Could you check a few things on this model? Use its own coordinates, in mm. A direction names the side the tool comes from. Give positions to 0.01 mm unless a question says otherwise; leave off trailing zeros. Order: outer loops, then holes, each group sorted by start corner. A loop starts at its lowest first (then second) coordinate and runs counter-clockwise, first axis right, second up. Notation, with made-up numbers: (77, 37) - (86, 37) arc R10 cw to (86, 43) - close; hole circle Ø6 at (60.25, -13). An arc over 180 degrees is marked (long way). Put each result on its own line as item: value.
from build123d import *

# Parameters (mm, degrees)
F0_W     = 41.148
F0_H     = 61.214
F1_DEPTH = 1.3
F2_R     = 1
F3_DEPTH = 1.3
F4_DEPTH = 4.5
F2_W     = 10.16
F2_H     = 1.5257
F5_DEPTH = 10.5
F2_H_2   = 4.445
F2_W_2   = 5.08
F6_DEPTH = 3.5
F2_H_3   = 1.905
F7_DEPTH = 11.5
F2_W_3   = 12.7
F8_DEPTH = 7.2


with BuildPart() as f1:
    # F0 (on Top) → F1 (new body)
    with BuildSketch(Plane.XY):
        Rectangle(F0_W, F0_H)
    extrude(amount=F1_DEPTH)

    # F2 (on face) → F3 (cut, through all)
    with BuildSketch(Plane.XY.offset(1.3)):
        with Locations((-18.034, 17.145)):
            Circle(F2_R)
        with Locations((18.034, 27.305)):
            Circle(F2_R)
        with Locations((18.034, -28.575)):
            Circle(F2_R)
    extrude(amount=-F3_DEPTH, mode=Mode.SUBTRACT)

    # F2 (on face) → F4 (join)
    with BuildSketch(Plane.XY.offset(1.3)):
        with BuildLine():
            ThreePointArc((-18.034, -4.826), (-17.399, -5.461), (-18.034, -6.096))
            Line((-18.034, -6.096), (-18.034, -8.255))
            Line((-18.034, -8.255), (19.05, -8.255))
            Line((19.05, -8.255), (19.05, -2.667))
            Line((19.05, -2.667), (-18.034, -2.667))
            Line((-18.034, -2.667), (-18.034, -4.826))
        make_face()
        with BuildLine():
            Line((14.224, 3.556), (14.224, 9.398))
            Line((14.224, 9.398), (-6.096, 9.398))
            Line((-6.096, 9.398), (-6.096, 7.493))
            ThreePointArc((-6.096, 7.493), (-5.08, 6.477), (-6.096, 5.461))
            Line((-6.096, 5.461), (-6.096, 3.556))
            Line((-6.096, 3.556), (14.224, 3.556))
        make_face()
        with BuildLine():
            Line((-1.016, -14.478), (-1.016, -20.32))
            Line((-1.016, -20.32), (19.304, -20.32))
            Line((19.304, -20.32), (19.304, -18.415))
            ThreePointArc((19.304, -18.415), (18.288, -17.399), (19.304, -16.383))
            Line((19.304, -16.383), (19.304, -14.478))
            Line((19.304, -14.478), (-1.016, -14.478))
        make_face()
    extrude(amount=F4_DEPTH)

    # F2 (on face) → F5 (join)
    with BuildSketch(Plane.XY.offset(1.3)):
        with Locations((-12.7211, 28.81415)):
            Rectangle(F2_W, F2_H)
        Polygon((-7.6411, 28.0513), (-17.8011, 28.0513), (-17.8011, 27.5683), (-17.8011, 23.5715), (-17.8011, 23.0791), (-7.6411, 23.0791), (-7.6411, 23.5715), (-7.6411, 27.5683), align=None)
        with BuildLine():
            ThreePointArc((-15.2611, 27.467), (-13.3461, 25.552), (-15.2611, 23.637))
            ThreePointArc((-15.2611, 23.637), (-17.1761, 25.552), (-15.2611, 27.467))
        make_face(mode=Mode.SUBTRACT)
        with BuildLine():
            ThreePointArc((-10.1811, 27.467), (-8.2661, 25.552), (-10.1811, 23.637))
            ThreePointArc((-10.1811, 23.637), (-12.0961, 25.552), (-10.1811, 27.467))
        make_face(mode=Mode.SUBTRACT)
    extrude(amount=F5_DEPTH)

    # F2 (on face) → F6 (join)
    with BuildSketch(Plane.XY.offset(1.3)):
        with Locations((7.874, 24.8285)):
            Rectangle(F2_W, F2_H_2)
        with Locations((-2.54, 17.5895)):
            Rectangle(F2_W_2, F2_H_2)
        with Locations((-13.208, -17.0815)):
            Rectangle(F2_W, F2_H_2)
    extrude(amount=F6_DEPTH)

    # F2 (on face) → F7 (join)
    with BuildSketch(Plane.XY.offset(1.3)):
        with Locations((7.874, 28.0035)):
            Rectangle(F2_W, F2_H_3)
        with Locations((-2.54, 14.4145)):
            Rectangle(F2_W_2, F2_H_3)
        with Locations((-13.208, -13.9065)):
            Rectangle(F2_W, F2_H_3)
    extrude(amount=F7_DEPTH)

    # F2 (on face) → F8 (join)
    with BuildSketch(Plane.XY.offset(1.3)):
        with Locations((9.144, 15.6845)):
            Rectangle(F2_W_3, F2_H_2)
        with Locations((9.144, 18.8595)):
            Rectangle(F2_W_3, F2_H_3)
        with Locations((8.382, -25.5905)):
            Rectangle(F2_W_3, F2_H_2)
        with Locations((8.382, -28.7655)):
            Rectangle(F2_W_3, F2_H_3)
    extrude(amount=F8_DEPTH)


solid = f1.part
1) I'm going to push flat-ended pins straight in: pin 1 (6 mm diameter, centred on x = 0.5, z = 10, fed in from +Y); pin 2 (2.5 mm diameter, centred on x = -10.18, y = 25.55, fed in from -Z); pin 3 (2 mm diameter, centred on y = -17.5, z = 4.5, fed in from -X); pin 4 (2 mm diameter, centred on x = 6, y = 25, fed in from +Z). Where does each tip first touch, or does it pass through?
Filled in:
pin 1: stops at y = 28.96
pin 2: stops at z = 0
pin 3: stops at x = -18.29
pin 4: stops at z = 4.8
2) Suppose I cut it at D-D, the plane y = -17.5. List the corners of the cut face in (x, z) for me, and give its area (3 significant figures).
Filled in:
outline: (-20.57, 0) - (20.57, 0) - (20.57, 1.3) - (18.29, 1.3) - (18.29, 5.8) - (-1.02, 5.8) - (-1.02, 1.3) - (-8.13, 1.3) - (-8.13, 4.8) - (-18.29, 4.8) - (-18.29, 1.3) - (-20.57, 1.3) - close
area: 176 mm^2
3) We'd pull the mould along Y, two halves only. Please class faces 1 (the cylindrical face through (-17.08, 17.45, 0.66)), 2 (the flat face through (-13, -14.859, 9)), 3 (the flat face through (-13, 29.577, 6)), 4 (the flat face through (8, -26, 8.5)): pulls with the +Y half, pulls with the -Y half, needs draft (parallel to the pull), parting line crosses it, or undercut.
Filled in:
face 1: undercut
face 2: pulls with the -Y half
face 3: pulls with the +Y half
face 4: needs draft
4) Which directions (+Z, -Z, +X, -X, +Y, -Y) give clear straight access to the entire face, cutting with the end or side of a thin tool? Please do faces 5 (the flat face through (-6.096, 8, 4)), 6 (the flat face through (4, 9.398, 4)), 7 (the flat face through (8, 28.956, 7)), 8 (the flat face through (-10, 26, 1.3)).
Filled in:
face 5: +Z, -X, +Y
face 6: +Z, +X, -X
face 7: +Z, +X, +Y
face 8: +Z
5) If I drill on line 1 (Y direction, x = 4.5, z = 5) (3 decimals); line 2 (Y direction, x = 5.5, z = 2) (3 decimals); line 3 (Y direction, x = 2.5, z = 5.75) (3 decimals), over which ranges is the centre line in solid material (lowest first)? Write a range as [from, to].
Filled in:
line 1: y = [-29.718, -23.368], [-20.32, -14.478], [-8.255, -2.667], [3.556, 9.398], [13.462, 19.812], [27.051, 28.956]
line 2: y = [-29.718, -23.368], [-20.32, -14.478], [-8.255, -2.667], [3.556, 9.398], [13.462, 19.812], [22.606, 28.956]
line 3: y = [-29.718, -23.368], [-20.32, -14.478], [-8.255, -2.667], [3.556, 9.398]
6) Suppose I cut it at B-B, the plane z = 7.75. List the corners of the cut face in (x, y) for me (3 decimals), and give its area (3 significant figures).
Filled in:
outline: (-18.288, -14.859) - (-8.128, -14.859) - (-8.128, -12.954) - (-18.288, -12.954) - close; (-17.801, 23.079) - (-7.641, 23.079) - (-7.641, 29.577) - (-17.801, 29.577) - close; (-5.08, 13.462) - (0, 13.462) - (0, 15.367) - (-5.08, 15.367) - close; (2.032, -29.718) - (14.732, -29.718) - (14.732, -23.368) - (2.032, -23.368) - close; (2.794, 13.462) - (15.494, 13.462) - (15.494, 19.812) - (2.794, 19.812) - close; (2.794, 27.051) - (12.954, 27.051) - (12.954, 28.956) - (2.794, 28.956) - close; hole circle Ø3.83 at (-15.261, 25.552); hole circle Ø3.83 at (-10.181, 25.552)
area: 253 mm^2
7) Suppose I cut it at C-C, the plane z = 10.5. List the corners of the cut face in (x, y) for me (3 decimals).
Filled in:
outline: (-18.288, -14.859) - (-8.128, -14.859) - (-8.128, -12.954) - (-18.288, -12.954) - close; (-17.801, 23.079) - (-7.641, 23.079) - (-7.641, 29.577) - (-17.801, 29.577) - close; (-5.08, 13.462) - (0, 13.462) - (0, 15.367) - (-5.08, 15.367) - close; (2.794, 27.051) - (12.954, 27.051) - (12.954, 28.956) - (2.794, 28.956) - close; hole circle Ø3.83 at (-15.261, 25.552); hole circle Ø3.83 at (-10.181, 25.552)
